```python
from build123d import *

# Parameters (mm, degrees)
SKETCH2_W          = 0.508
SKETCH2_H          = 41.656
CUT_EXTRUDE1_REACH = 61.086
SKETCH3_R          = 1.651
CIRPATTERN1_COUNT  = 6


with BuildPart() as part:
    # Sketch2 → Revolve1 (revolve)
    with BuildSketch(Plane.XY, mode=Mode.PRIVATE) as revolve1_sk:
        with Locations((-0.254, 20.828)):
            Rectangle(SKETCH2_W, SKETCH2_H)
        with BuildLine():
            ThreePointArc((0, 41.656), (1.7653, 39.8907), (3.5306, 41.656))
            Line((3.5306, 41.656), (3.5306, 0))
            Line((3.5306, 0), (0, 0))
            Line((0, 0), (0, 41.656))
        make_face()
        with Locations((3.7846, 20.828)):
            Rectangle(SKETCH2_W, SKETCH2_H)
    revolve(revolve1_sk.sketch.rotate(Axis((0, 0, 0), (1, 0, 0)), 90), axis=Axis((0, 0, 0), (1, 0, 0)))

    # Sketch3 → Cut-Extrude1 (cut, up to next)
    with BuildSketch(Plane(origin=(-0.508, 0, 0), x_dir=(0, 0, -1), z_dir=(1, 0, 0)), mode=Mode.PRIVATE) as cut_extrude1_sk1:
        with BuildLine():
            ThreePointArc((6.764649654, 21.414174788), (-0.091034511, 22.457049662), (-6.938038467, 21.358627977))
            Line((-6.938038467, 21.358627977), (-3.409234604, 8.509))
            Line((-3.409234604, 8.509), (3.48250762, 8.509))
            Line((3.48250762, 8.509), (6.764649654, 21.414174788))
        make_face()
    cut_extrude1_tool1 = extrude(cut_extrude1_sk1.sketch, amount=CUT_EXTRUDE1_REACH, mode=Mode.PRIVATE) & part.part
    # Sketch3 → Cut-Extrude1 (cut, up to next)
    with BuildSketch(Plane(origin=(-0.508, 0, 0), x_dir=(0, 0, -1), z_dir=(1, 0, 0)), mode=Mode.PRIVATE) as cut_extrude1_sk2:
        with BuildLine():
            Line((6.764649654, 21.414174788), (3.48250762, 8.509))
            Line((3.48250762, 8.509), (15.057941963, 33.332599056))
            ThreePointArc((15.057941963, 33.332599056), (0.03320673, 36.575984926), (-14.997392963, 33.359885796))
            Line((-14.997392963, 33.359885796), (-3.409234604, 8.509))
            Line((-3.409234604, 8.509), (-6.938038467, 21.358627977))
            ThreePointArc((-6.938038467, 21.358627977), (-0.091034511, 22.457049662), (6.764649654, 21.414174788))
        make_face()
    cut_extrude1_tool2 = extrude(cut_extrude1_sk2.sketch, amount=CUT_EXTRUDE1_REACH, mode=Mode.PRIVATE) & part.part
    # Sketch3 → Cut-Extrude1 (cut, up to next)
    with BuildSketch(Plane(origin=(-0.508, 0, 0), x_dir=(0, 0, -1), z_dir=(1, 0, 0)), mode=Mode.PRIVATE) as cut_extrude1_sk3:
        Polygon((6.892407514, 0), (3.446203757, 5.969), (-3.446203757, 5.969), (-6.892407514, 0), (-3.446203757, -5.969), (3.446203757, -5.969), align=None)
        Circle(SKETCH3_R, mode=Mode.SUBTRACT)
    cut_extrude1_tool3 = extrude(cut_extrude1_sk3.sketch, amount=CUT_EXTRUDE1_REACH, mode=Mode.PRIVATE) & part.part
    # Sketch3 → Cut-Extrude1 (cut, up to next)
    with BuildSketch(Plane(origin=(-0.508, 0, 0), x_dir=(0, 0, -1), z_dir=(1, 0, 0)), mode=Mode.PRIVATE) as cut_extrude1_sk4:
        Circle(SKETCH3_R)
    cut_extrude1_tool4 = extrude(cut_extrude1_sk4.sketch, amount=CUT_EXTRUDE1_REACH, mode=Mode.PRIVATE) & part.part
    cut_extrude1_1 = cut_extrude1_tool1.solids().sort_by_distance((-0.508, 16.082461, 0.033427))[0]
    add(cut_extrude1_1, mode=Mode.SUBTRACT)
    cut_extrude1_2 = cut_extrude1_tool2.solids().sort_by_distance((-0.508, 28.201859, -0.056512))[0]
    add(cut_extrude1_2, mode=Mode.SUBTRACT)
    cut_extrude1_3 = cut_extrude1_tool3.solids().sort_by_distance((-0.508, 2.893322, -5.011381))[0]
    add(cut_extrude1_3, mode=Mode.SUBTRACT)
    cut_extrude1_4 = cut_extrude1_tool4.solids().sort_by_distance((-0.508, 0, 0))[0]
    add(cut_extrude1_4, mode=Mode.SUBTRACT)
    cut_extrude1 = cut_extrude1_1 + cut_extrude1_2 + cut_extrude1_3 + cut_extrude1_4  # Cut-Extrude1 as one shape, for the pattern or mirror that repeats it

    # CirPattern1: Cut-Extrude1 ×6 about axis
    cirpattern1_axis = Axis((0, 0, 0), (1, 0, 0))
    for i in range(1, CIRPATTERN1_COUNT):
        add(cut_extrude1.rotate(cirpattern1_axis, i * 360 / CIRPATTERN1_COUNT), mode=Mode.SUBTRACT)


solid = part.part
```
Geometry: final body of the model. Coordinates: model frame, mm. Round coordinates to 2 decimals unless told otherwise and drop trailing zeros. Answer in a Markdown table with one row per item. Add a question column.
(1) Draft query along Y for faces 1 (the face through (1.7, 4.2, 7.4)), 2 (the face through (-0.25, -12.512, 39.732)). Return one class per face: pulls with the +Y half, pulls with the -Y half, needs draft (parallel to the pull), parting line crosses it, or undercut.
(2) Ray query, L1, parallel to Z at x = 3.3, y = -23.5; L2, parallel to Y at x = 1.8, z = 1; L3, parallel to Y at x = 1.05, z = -8.5. Return the intervals inside material, ascending.
(3) Contact query for flat-ended pins moving along their axis: pin 1 (1.4 mm diameter, centred on x = 1.5, z = -0.5, fed in from -Y) (3 decimals); pin 2 (1.4 mm diameter, centred on x = 2, z = -1, fed in from +Y). Output: stop coordinate, or through.
(4) Cut plane B-B, the plane x = 1.05. Give the number of separate pieces and of enclosed holes in the cut face, then the cut area to 3 significant figures.
Established:
| question | item | result |
|---|---|---|
| 1 | face 1 | undercut |
| 1 | face 2 | parting line crosses it |
| 2 | L1 | -33.33 to -28.03, -16.99 to -10.4, 10.47 to 17.07, 28.03 to 33.33 |
| 2 | L2 | -39.88 to -36.56, -8.51 to -5.97, 5.97 to 8.51, 36.56 to 39.88 |
| 2 | L3 | -39.13 to -35.57, -19.43 to -11.37, -2.3 to 2.3, 11.26 to 19.27, 35.57 to 39.13 |
| 3 | pin 1 | y = -40.175 |
| 3 | pin 2 | y = 40.15 |
| 4 | separate pieces | 1 |
| 4 | enclosed holes | 7 |
| 4 | area | 1,770 mm² |
